Check sheet for the modelled part. Datum: model origin and axes. Units: mm. Face numbers are marked on the shaded views. A direction names the side the tool comes from. Round coordinates to 2 decimals unless told otherwise and drop trailing zeros. Write each loop counter-clockwise with the first axis right and the second up, starting at its lowest first coordinate (ties: lowest second). Pieces come first, ordered by that corner, then holes. Notation, with made-up numbers: M -16.5,40.25 L 39.5,40.25 A22 cw 39.5,47.25 Z; hole C 4,-25.75 d2. An arc over 180 degrees is marked long. One line per item, written item: value.
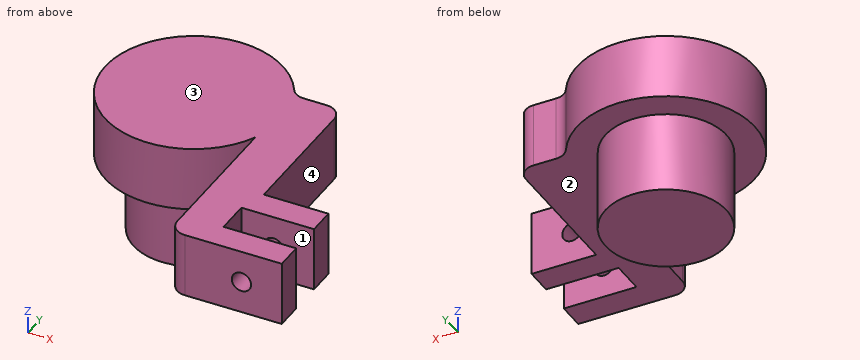
from build123d import *

# Parameters (mm, degrees)
BOSS_EXTRU_1_DEPTH      = 8
ENL_V_MAT_EXTRU_1_REACH = 45.749
ESQUISSE2_R             = 1
D_GAGEMENT_M21_D        = 2.4
D_GAGEMENT_M21_DEPTH    = 11
D_GAGEMENT_M21_TIP      = 0.721032743
CONG_1_R                = 2
ESQUISSE6_R             = 7.5
BOSS_EXTRU_3_DEPTH      = 10


with BuildPart() as part:
    # Esquisse1 → Boss.-Extru.1 (new body)
    with BuildSketch(Plane.XY):
        with BuildLine():
            Line((21, -6.417424305), (27, -6.417424305))
            Line((27, -6.417424305), (27, -25))
            Line((27, -25), (35, -25))
            Line((35, -25), (35, -28.4))
            Line((35, -28.4), (26, -28.4))
            Line((26, -28.4), (26, -32.6))
            Line((26, -32.6), (35, -32.6))
            Line((35, -32.6), (35, -36))
            Line((35, -36), (21, -36))
            Line((21, -36), (21, -15.582575695))
            ThreePointArc((21, -15.582575695), (0, -11), (21, -6.417424305))
        make_face()
    extrude(amount=BOSS_EXTRU_1_DEPTH)

    # Enlèv. mat.-Extru.1: up to this face of the body (flat: up to its plane)
    enl_v_mat_extru_1_end = Plane(part.part.faces().sort_by_distance((28, -36, 4))[0])
    # Esquisse2 → Enlèv. mat.-Extru.1 (cut, up to the picked face)
    with BuildSketch(Plane(origin=(0, -25, 0), x_dir=(1, 0, 0), z_dir=(0, 1, 0)), mode=Mode.PRIVATE) as enl_v_mat_extru_1_sk1:
        with Locations(Location((30, -4, 0), (0, 0, 270))):
            Circle(ESQUISSE2_R)
    enl_v_mat_extru_1_tool1 = split(extrude(enl_v_mat_extru_1_sk1.sketch, amount=-ENL_V_MAT_EXTRU_1_REACH, mode=Mode.PRIVATE), bisect_by=enl_v_mat_extru_1_end, keep=Keep.BOTH, mode=Mode.PRIVATE)
    add(enl_v_mat_extru_1_tool1.solids().sort_by(Axis((30, -25, 4), (0, -1, 0)))[0], mode=Mode.SUBTRACT)

    # Dégagement M21
    with Locations(Plane(origin=(0, -25, 0), x_dir=(1, 0, 0), z_dir=(0, 1, 0))):
        with Locations((30, -4)):
            Hole(D_GAGEMENT_M21_D / 2, depth=D_GAGEMENT_M21_DEPTH)
            with Locations((0, 0, -(D_GAGEMENT_M21_DEPTH + D_GAGEMENT_M21_TIP / 2))):  # 118° drill point
                Cone(0, D_GAGEMENT_M21_D / 2, D_GAGEMENT_M21_TIP, mode=Mode.SUBTRACT)

    # Congé1
    cong_1_edges = [part.edges().sort_by_distance(p)[0] for p in [
        (21, -36, 4),
        (21, -6.417424305, 4),
        (27, -6.417424305, 4),
    ]]
    fillet(cong_1_edges, radius=CONG_1_R)

    # Esquisse6 → Boss.-Extru.3 (add)
    with BuildSketch(Plane(origin=(0, 0, 0), x_dir=(-1, 0, 0), z_dir=(0, 0, -1))):
        with Locations(Location((-11, -11, 0), (0, 0, 180))):
            Circle(ESQUISSE6_R)
    extrude(amount=BOSS_EXTRU_3_DEPTH)


solid = part.part
Q1. Scan lines: line 1 (Z direction, x = 30, y = -35.2); line 2 (X direction, y = -26.15, z = 4); line 3 (X direction, y = -25.5, z = 5). Record each from-to range of solid material in increasing order. Write a range as [from, to].
Completed:
line 1: [0, 2.8], [5.2, 8]
line 2: [21, 28.8], [31.2, 35]
line 3: [21, 29.34], [30.66, 35]
Q2. Sectioned sample at A-A on z = 4. Enter the section's corners in (x, y), and give its area (3 significant figures).
Completed:
outline: M 20.49,-5.43 A11 ccw long 21,-15.58 L 21,-34 A2 ccw 23,-36 L 28.8,-36 L 28.8,-32.6 L 26,-32.6 L 26,-28.4 L 28.8,-28.4 L 28.8,-25 L 27,-25 L 27,-8.42 A2 ccw 25,-6.42 L 22.21,-6.42 A2 cw Z; M 31.2,-36 L 35,-36 L 35,-32.6 L 31.2,-32.6 Z; M 31.2,-28.4 L 35,-28.4 L 35,-25 L 31.2,-25 Z
area: 584 mm^2
Q3. Sectioned sample at D-D on z = 7. Enter the section's corners in (x, y).
Completed:
outline: M 20.49,-5.43 A11 ccw long 21,-15.58 L 21,-34 A2 ccw 23,-36 L 35,-36 L 35,-32.6 L 26,-32.6 L 26,-28.4 L 35,-28.4 L 35,-25 L 27,-25 L 27,-8.42 A2 ccw 25,-6.42 L 22.21,-6.42 A2 cw Z
Q4. Sectioned sample at B-B on x = 30. Enter the section's corners in (y, z).
Completed:
outline: M -36,0 L -32.6,0 L -32.6,2.8 L -36,2.8 Z; M -36,5.2 L -32.6,5.2 L -32.6,8 L -36,8 Z; M -28.4,0 L -25,0 L -25,2.8 L -28.4,2.8 Z; M -28.4,5.2 L -25,5.2 L -25,8 L -28.4,8 Z
Q5. Access from +Z, -Z, +X, -X, +Y, -Y to the whole of each face (thin tool, end or side, straight path). Record for the marked faces 1, 2, 3 and 4.
Completed:
face 1: +Z, -Z, +X
face 2: -Z
face 3: +Z, +X, -X, +Y, -Y
face 4: +Z, -Z, +X, +Y
Q6. Depth check by flat-ended pin: P1, Ø1, axis at y = -10.5, z = -8, coming from the +X side; P2, Ø10.5, axis at x = 22.5, y = -24.5, coming from the -Z side; P3, Ø4, axis at x = 29.5, z = 3.5, coming from the +Y side. Enter the tip coordinate at first touch or a pass-through.
Completed:
P1: x = 18.5
P2: z = 0
P3: y = -25
Q7. Sectioned sample at C-C on y = -27.5. Enter the section's corners in (x, z).
Completed:
outline: M 21,0 L 35,0 L 35,8 L 21,8 Z; hole C 30,4 d2.4
